```python
from build123d import *

# Parameters (mm, degrees)
SKETCH1_R           = 15
FACE_2_DEPTH        = 5
L_START             = -5
L_LINK_DEPTH        = 5
SKETCH3_R           = 1
FIXING_SCREWS_DEPTH = 83.006097334


with BuildPart() as part:
    # Sketch1 → face 2 (new body)
    with BuildSketch(Plane.XY):
        Circle(SKETCH1_R)
    extrude(amount=FACE_2_DEPTH)

    # Sketch2 → L link (add)
    with BuildSketch(Plane.XY.offset(L_START)):
        with BuildLine():
            ThreePointArc((0, -15), (-15, 0), (0, 15))
            Line((0, 15), (-80, 15))
            Line((-80, 15), (-80, -15))
            Line((-80, -15), (0, -15))
        make_face()
        with BuildLine():
            ThreePointArc((15, 0), (10.606601718, 10.606601718), (0, 15))
            Line((0, 15), (0, -15))
            ThreePointArc((0, -15), (10.606601718, -10.606601718), (15, 0))
        make_face()
        with BuildLine():
            Line((0, -15), (0, 15))
            ThreePointArc((0, 15), (-15, 0), (0, -15))
        make_face()
    l_link = extrude(amount=L_LINK_DEPTH)

    # Sketch3 → fixing screws (cut, through all)
    with BuildSketch(Plane.XY.offset(5)):
        with Locations((0, 5)):
            Circle(SKETCH3_R)
        with Locations((5, 0)):
            Circle(SKETCH3_R)
        with Locations((0, -5)):
            Circle(SKETCH3_R)
        with Locations((-5, 0)):
            Circle(SKETCH3_R)
    extrude(amount=-FIXING_SCREWS_DEPTH, mode=Mode.SUBTRACT)

    # Mirror2: L link across plane
    add(l_link.mirror(Plane(origin=(-40, 0, -40), x_dir=(-0.7071067811865478, 0, 0.7071067811865472), z_dir=(0.7071067811865475, 0, 0.7071067811865477))))


solid = part.part
```
The model under review builds one solid part; all positions refer to its coordinate system, in mm. A direction names the side the tool comes from. Give positions to 0.01 mm unless a question says otherwise; leave off trailing zeros. Write each loop counter-clockwise with the first axis right and the second up, starting at its lowest first coordinate (ties: lowest second). Pieces come first, ordered by that corner, then holes. Notation, with made-up numbers: M 13.5,7 L 57.5,7 A24 ccw 57.5,30 Z; hole C -36.75,-7.5 d5. An arc over 180 degrees is marked long. Write item = value, one per line. Start each with the question number.
Q1. We need section C-C (z = -73.5). State the section outline as (x, y) points.
Q2. Machinability: for faces 1 (the face through (-75, 0, -49)), 2 (the face through (-80, 0, -48)), which of the approach directions +Z, -Z, +X, -X, +Y, -Y give a long, thin tool a straight path to every point of the face, cutting with its end or side? Answer none if there is none.
Q3. We need section D-D (x = -60.5). State the section outline as (y, z) points, plus the area to 3 significant figures.
Q4. Clearance check with flat-ended pins moving along their axes: pin 1 (3 mm diameter, centred on x = 0, y = -5, fed in from -Z); pin 2 (2 mm diameter, centred on x = -47, y = -11.5, fed in from +Z); pin 3 (6 mm diameter, centred on y = -10.5, z = -24, fed in from +X). State where each tip first meets the part, or that it passes through.
Q5. We need section A-A (y = 10.75). State the section outline as (x, z) points, plus the area to 3 significant figures.
Q6. For line 1 (Y direction, x = 0, z = 0); line 2 (Y direction, x = -5, z = -1); line 3 (X direction, y = -11, z = -85), list the stretches that pass through material, from the lowest coordinate up.
Q7. We need section B-B (x = -13.5). State the section outline as (y, z) points, plus the area to 3 significant figures.
Result set:
q1.outline = M -80,-15 L -75,-15 L -75,15 L -80,15 Z
q2.face_1 = -Z, +X, +Y, -Y
q2.face_2 = +Z, -Z, -X, +Y, -Y
q3.outline = M -15,-5 L 15,-5 L 15,0 L -15,0 Z
q3.area = 150 mm2
q4.pin_1 = -5
q4.pin_2 = 0
q4.pin_3 = -75
q5.outline = M -80,-90.46 L -75,-90.46 L -75,-5 L 10.46,-5 L 10.46,5 L -10.46,5 L -10.46,0 L -80,0 Z
q5.area = 984 mm2
q6.line_1 = -15 to -6, -4 to 4, 6 to 15
q6.line_2 = -15 to -1, 1 to 15
q6.line_3 = -80 to -75
q7.outline = M -15,-5 L 15,-5 L 15,0 L 6.54,0 L 6.54,5 L -6.54,5 L -6.54,0 L -15,0 Z
q7.area = 215 mm2
